The model under review builds one solid part; all positions refer to its coordinate system, in mm. Give positions to 0.01 mm unless a question says otherwise; leave off trailing zeros. Loops run counter-clockwise (first coordinate to the right, second up) from the corner with the lowest first, then second, coordinate; pieces in that order, holes last. Notation, with made-up numbers: (2.5, 51.25) - (47.5, 51.25) arc R31 ccw to (47.5, 76.25) - close; hole circle Ø7 at (2.5, 79). An arc over 180 degrees is marked (long way). Return JSON: item names as keys, results as strings. Group by question number.
from build123d import *

# Parameters (mm, degrees)
SWEEP1_PROFILE_R     = 6.35
CUT_SWEEP2_START     = 168.275
CUT_SWEEP2_OUTLINE_W = 16
CUT_SWEEP2_OUTLINE_H = 42
CUT_SWEEP2_DEPTH     = 73.999175886


# Read off the part's stored shape, not the designer's step: Cut-Sweep2
with BuildPart() as part:
    # Sweep1: sweep along a path in Sketch1
    with BuildLine(Plane(origin=(0, 0, 0), x_dir=(1, 0, 0), z_dir=(0, 1, 0))) as sweep1_path:
        Line((0, 0), (59.58888407, 0))
        ThreePointArc((59.58888407, 0), (72.820875208, -1.15764922), (85.650818991, -4.595422296))
        Line((85.650818991, -4.595422296), (168.497770272, -34.749246562))
        Line((168.497770272, -34.749246562), (240.102347976, -60.811181483))
    # Sweep1 profile (on start of the path) → Sweep1 (sweep)
    with BuildSketch(Plane(origin=(0, 0, 0), x_dir=(0, 0, 1), z_dir=(1, 0, 0))):
        Circle(SWEEP1_PROFILE_R)
    sweep1 = sweep(path=sweep1_path.line)

    # Cut-Sweep2 outline → Cut-Sweep2 (cut)
    with BuildSketch(Plane.YZ.offset(CUT_SWEEP2_START)):
        with Locations((0, 47)):
            Rectangle(CUT_SWEEP2_OUTLINE_W, CUT_SWEEP2_OUTLINE_H)
    cut_sweep2 = extrude(amount=CUT_SWEEP2_DEPTH, mode=Mode.SUBTRACT)

    # Mirror1: Sweep1, Cut-Sweep2 across plane
    add(sweep1.mirror(Plane(origin=(0, 0, 0), x_dir=(0, 0, 1), z_dir=(1, 0, 0))))
    add(cut_sweep2.mirror(Plane(origin=(0, 0, 0), x_dir=(0, 0, 1), z_dir=(1, 0, 0))), mode=Mode.SUBTRACT)


solid = part.part
Item 1: For P1, Ø2, axis at x = 87, z = 8, coming from the -Y side; P2, Ø3, axis at x = 119.5, y = 3, coming from the +Z side; P3, Ø1, axis at x = -132, y = 4, coming from the -Z side, all flat-tipped, find the tip position at first contact; note any pin that passes through.
Item 2: Take a section at B-B (x = 50.5). State the section outline as (y, z) points.
Item 3: Take a section at A-A (y = -3.75). State the section outline as (x, z) points (1 decimal), then the cut area to 3 significant figures.
Item 4: For L1, parallel to Z at x = 36, y = -1; L2, parallel to Z at x = -39.5, y = -1.75; L3, parallel to Y at x = -52, z = -3.5, list the stretches that pass through material, from the lowest coordinate up. Write a range as from..to.
Check sheet entries:
{
 "1": {"P1": "stops at y = -6.11", "P2": "stops at z = 23.74", "P3": "stops at z = 15.78"},
 "2": {"outline": "circle Ø12.7 at (0, 0)"},
 "3": {"outline": "(-168.3, 29.2) - (-87.4, -0.2) arc R81.3 ccw to (-59.6, -5.1) - (59.6, -5.1) arc R81.3 ccw to (87.4, -0.2) - (168.3, 29.2) - (168.3, 40.1) - (83.9, 9.4) arc R71.1 cw to (59.6, 5.1) - (-59.6, 5.1) arc R71.1 cw to (-83.9, 9.4) - (-168.3, 40.1) - close", "area": "3,570 mm^2"},
 "4": {"L1": "z = -6.27..6.27", "L2": "z = -6.1..6.1", "L3": "y = -5.3..5.3"}
}
